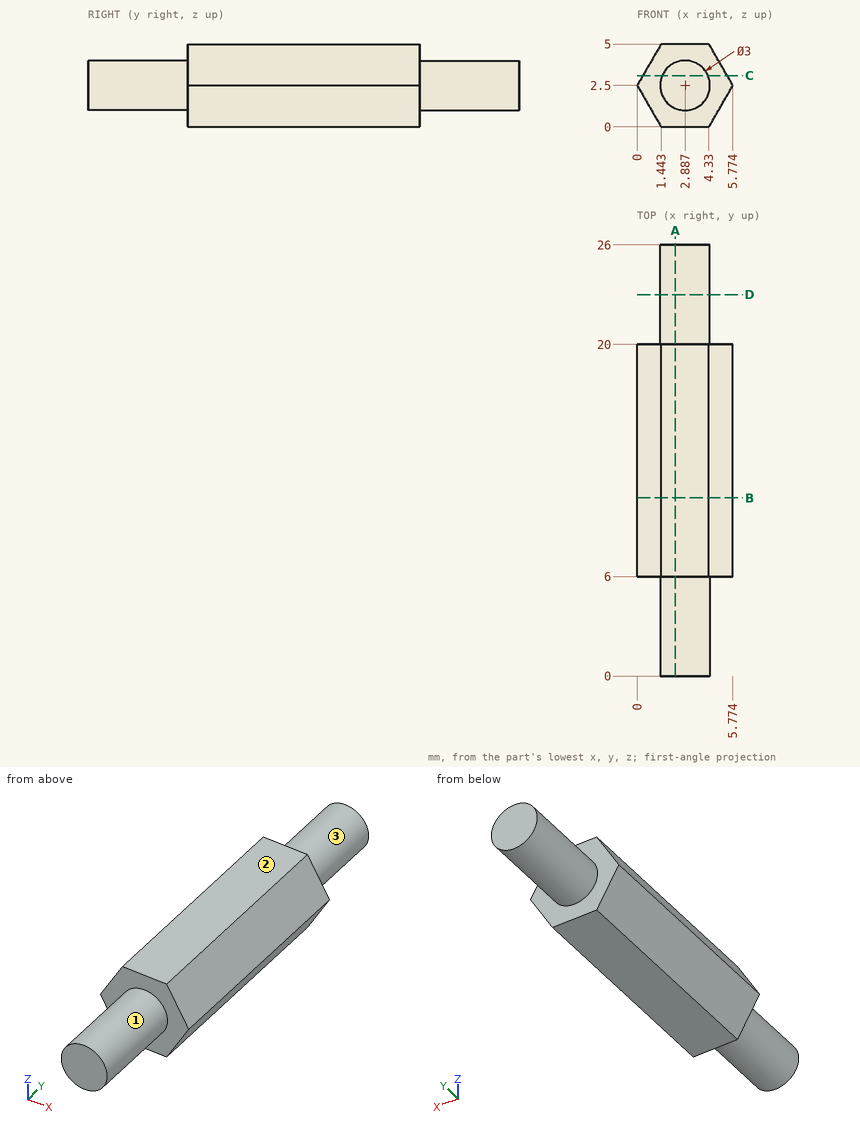
The drawing under review shows one solid part. Ordinate dimensions are in mm from its lowest x, y, z. A direction names the side the tool comes from. Give positions to 0.01 mm unless a question says otherwise; leave off trailing zeros. Loops run counter-clockwise (first coordinate to the right, second up) from the corner with the lowest first, then second, coordinate; pieces in that order, holes last. Notation, with made-up numbers: M 43,65.5 L 88,65.5 A12 cw 88,82.5 Z; hole C -20.5,87 d2. An arc over 180 degrees is marked long. Return JSON: item names as keys, results as strings. Group by question number.
Item 1: We need section A-A (x = 2.3). Give the boundary of the cut face in (y, z), and give its area (3 significant figures).
Item 2: We need section D-D (y = 23). Give the boundary of the cut face in (x, z).
Item 3: For probe 1 along Y at (x, z) = (1.2, 4.5); probe 2 along X at (y, z) = (8, 3.7); probe 3 along X at (y, z) = (8.75, 0.55) (1 decimal), list the stretches that pass through material, from the lowest coordinate up.
Item 4: We need section B-B (y = 10.75). Give the boundary of the cut face in (x, z).
Item 5: Tool access review of the marked faces 1, 2 and 3: name each direction out of +Z, -Z, +X, -X, +Y, -Y from which nothing blocks a thin tool from reaching the whole face with its end or side.
Item 6: We need section C-C (z = 3.1). Give the boundary of the cut face in (x, y), and give its area (3 significant figures).
Output:
{
 "1": {"outline": "M 0,1.12 L 6,1.12 L 6,0 L 20,0 L 20,1.12 L 26,1.12 L 26,3.88 L 20,3.88 L 20,5 L 6,5 L 6,3.88 L 0,3.88 Z", "area": "103 mm^2"},
 "2": {"outline": "C 2.89,2.5 d3"},
 "3": {"probe 1": "y = 6 to 20", "probe 2": "x = 0.69 to 5.08", "probe 3": "x = 1.1 to 4.6"},
 "4": {"outline": "M 0,2.5 L 1.44,0 L 4.33,0 L 5.77,2.5 L 4.33,5 L 1.44,5 Z"},
 "5": {"face 1": "-Y", "face 2": "+Z, +X, -X, +Y, -Y", "face 3": "+Y"},
 "6": {"outline": "M 0.35,6 L 1.51,6 L 1.51,0 L 4.26,0 L 4.26,6 L 5.43,6 L 5.43,20 L 4.26,20 L 4.26,26 L 1.51,26 L 1.51,20 L 0.35,20 Z", "area": "104 mm^2"}
}
